```python
from build123d import *

# Parameters (mm, degrees)
F0_R      = 45
F3_DEPTH  = 35
F4_R      = 45
F2_R      = 32.5
F9_D      = 30
F10_D     = 8.5
F10_DEPTH = 45
F10_START = 0.2011441
F10_TIP   = 2.5536576309


# Not quite as in the source:
# - a fillet or chamfer that OpenCascade refuses, or shapes differently, is made with other operations: its cross-section is extruded or revolved along the edge and cut away or added


with BuildPart() as f3:
    # F0 (on Right) → F3 (new body)
    with BuildSketch(Plane.YZ):
        Circle(F0_R)
    extrude(amount=F3_DEPTH)

    # F4 (on face) → F5 section 0
    with BuildSketch(Plane.YZ.offset(35)):
        Circle(F4_R)
    # F2 (on offset) → F5 section 1
    with BuildSketch(Plane.YZ.offset(95)):
        Circle(F2_R)
    loft()

    # F9 (through all)
    with Locations(Plane.YZ.offset(95)):
        with Locations((0, 0)):
            Hole(F9_D / 2)

    # F10
    # its depths count from where the whole tool has entered the part; down to there all is cleared
    with Locations(Plane.XY.offset(45).offset(-F10_START)):
        with Locations((18, 0)):
            Hole(F10_D / 2, depth=F10_DEPTH)
            with Locations((0, 0, -(F10_DEPTH + F10_TIP / 2))):  # 118° drill point
                Cone(0, F10_D / 2, F10_TIP, mode=Mode.SUBTRACT)

    # F11: chamfer of 1.5 on 4 edges, made by hand

    # F11_s1 → F11_t2 (revolve, cut)
    with BuildSketch(Plane.XY):
        Polygon((93.8059313812, 32.7487642956), (95, 31.280293666), (95, 32.5), align=None)
    revolve(axis=Axis((95, 0, 0), (1, 0, 0)), mode=Mode.SUBTRACT)

    # F11_s3 → F11_t4 (revolve, cut)
    with BuildSketch(Plane.XY):
        Polygon((1.5, 45), (0, 43.5), (0, 45), align=None)
    revolve(axis=Axis((0, 0, 0), (1, 0, 0)), mode=Mode.SUBTRACT)

    # F11_s5 → F11_t6 (revolve, cut)
    with BuildSketch(Plane.XY):
        Polygon((0, 16.5), (1.5, 15), (0, 15), align=None)
    revolve(axis=Axis((0, 0, 0), (1, 0, 0)), mode=Mode.SUBTRACT)

    # F11_s7 → F11_t8 (revolve, cut)
    with BuildSketch(Plane.XY):
        Polygon((93.5, 15), (95, 16.5), (95, 15), align=None)
    revolve(axis=Axis((95, 0, 0), (1, 0, 0)), mode=Mode.SUBTRACT)


solid = f3.part
```
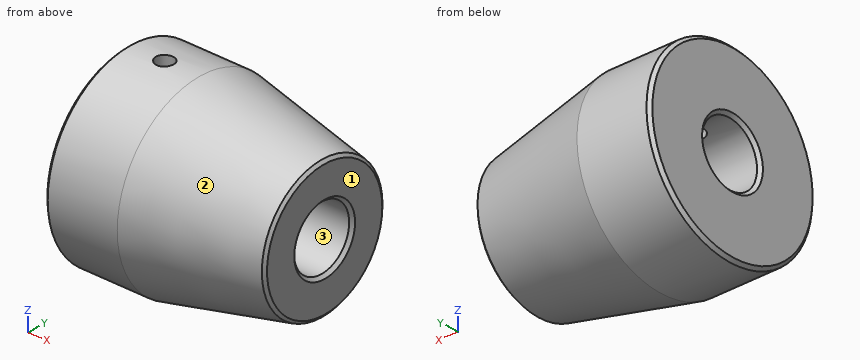
CAD build for the part. Positions are in the model's coordinates, mm. Face numbers are marked on the shaded views. Round coordinates to 2 decimals unless told otherwise and drop trailing zeros. Order: outer loops, then holes, each group sorted by start corner. A loop starts at its lowest first (then second) coordinate and runs counter-clockwise, first axis right, second up.
Item 1: Probe line 1 along X through (y, z) = (0, 27); line 2 along Y through (x, z) = (38, -8.5); line 3 along Y through (x, z) = (22, 3). List the from-to ranges inside material, lowest first.
Item 2: Mould opens along Y. For the marked faces 1, 2 and 3 say: pulls with the +Y half, pulls with the -Y half, needs draft (parallel to the pull), parting line crosses it, or undercut.
Item 3: Saw through at B-B on x = 18. Write the cut outline in (y, z), then the cut area to 3 significant figures.
Item 4: Saw through at D-D on x = 73. Write the cut outline in (y, z).
Item 5: Saw through at A-A on y = 0. Write the cut outline in (x, z).
Item 6: Saw through at C-C on x = 44. Write the cut outline in (y, z) (3 decimals).
Item 7: Pin check, flat tips, straight feed: pin 1 (3 mm diameter, centred on x = 67.5, z = 35.5, fed in from +Y); pin 2 (1 mm diameter, centred on x = 36.5, z = -24, fed in from +Y); pin 3 (1.5 mm diameter, centred on x = 72, z = 32.5, fed in from -Y). Stop position of each tip, or through.
Reported:
1. line 1: x = 0 to 13.75, 22.25 to 95
1. line 2: y = -43.55 to -12.36, 12.36 to 43.55
1. line 3: y = -44.9 to -14.7, 14.7 to 44.9
2. face 1: needs draft
2. face 2: parting line crosses it
2. face 3: undercut
3. outline: (-4.25, 14.39) - (-4.25, 44.8) arc R45 ccw (long way) to (4.25, 44.8) - (4.25, 14.39) arc R15 cw (long way) to start
3. area: 5,400 mm2
4. outline: circle Ø74.17 at (0, 0); hole circle Ø30 at (0, 0)
5. outline: (0, -43.5) - (1.5, -45) - (35, -45) - (93.81, -32.75) - (95, -31.28) - (95, -16.5) - (93.5, -15) - (1.5, -15) - (0, -16.5) - close; (0, 16.5) - (1.5, 15) - (13.75, 15) - (13.75, 45) - (1.5, 45) - (0, 43.5) - close; (22.25, 15) - (93.5, 15) - (95, 16.5) - (95, 31.28) - (93.81, 32.75) - (35, 45) - (22.25, 45) - close
6. outline: circle Ø86.25 at (0, 0); hole circle Ø30 at (0, 0)
7. pin 1: stops at y = 17.56
7. pin 2: stops at y = 38.03
7. pin 3: stops at y = -19.6
